Input: part model. Units: mm. Frame: model coordinates. A direction names the side the tool comes from. Give positions to 0.01 mm unless a question says otherwise; leave off trailing zeros. Order: outer loops, then holes, each group sorted by start corner. A loop starts at its lowest first (then second) coordinate and runs counter-clockwise, first axis right, second up. Notation, with made-up numbers: (11, 82) -> (68, 82) arc R20 ccw to (68, 106) -> close; hole circle Ø11 at (57.5, 73). An arc over 180 degrees is marked (long way). Use a Markdown table: item, result. Add a question column.
from build123d import *

# Parameters (mm, degrees)
SKETCH1_R           = 7.750000000000002
SKETCH1_R_2         = 2.7500000000000013
SKETCH1_R_3         = 7.749999999999997
SKETCH1_R_4         = 2.7499999999999973
BOSS_EXTRUDE1_DEPTH = 5
BOSS_EXTRUDE2_DEPTH = 5
BOSS_EXTRUDE3_DEPTH = 10
BOSS_EXTRUDE4_DEPTH = 5
FILLET1_R           = 5
SKETCH6_R           = 3.5
CUT_EXTRUDE1_DEPTH  = 5
CUT_EXTRUDE2_DEPTH  = 3
BOSS_EXTRUDE5_DEPTH = 3
FILLET2_R           = 10
BOSS_EXTRUDE6_DEPTH = 5
FILLET3_R           = 2


with BuildPart() as part:
    # Sketch1 → Boss-Extrude1 (new body)
    # profile 1 of 4: a face of its own
    with BuildSketch(Plane.XY):
        with BuildLine():
            ThreePointArc((-10.000000000000002, 33.49999999999998), (-17.75, 41.24999999999998), (-10, 48.99999999999998))
            Line((-10, 48.99999999999998), (-60.00000000000001, 48.99999999999998))
            Line((-60.00000000000001, 48.99999999999998), (-60, 33.49999999999997))
            Line((-60, 33.49999999999997), (-10, 33.49999999999998))
        make_face()
    # profile 2 of 4: a face of its own
    with BuildSketch(Plane.XY):
        with Locations((-10, 41.24999999999998)):
            Circle(SKETCH1_R)
        with Locations((-10, 41.24999999999998)):
            Circle(SKETCH1_R_2, mode=Mode.SUBTRACT)
    # profile 3 of 4: a face of its own
    with BuildSketch(Plane.XY):
        with Locations((-9.999999999999927, -41.24999999999999)):
            Circle(SKETCH1_R_3)
        with Locations((-9.999999999999927, -41.24999999999999)):
            Circle(SKETCH1_R_4, mode=Mode.SUBTRACT)
    # profile 4 of 4: a face of its own
    with BuildSketch(Plane.XY):
        with BuildLine():
            Line((-59.99999999999993, -48.999999999999986), (-9.999999999999927, -48.99999999999999))
            ThreePointArc((-9.999999999999929, -48.99999999999999), (-17.749999999999925, -41.24999999999999), (-9.999999999999927, -33.49999999999999))
            Line((-9.999999999999927, -33.49999999999999), (-59.99999999999993, -33.5))
            Line((-59.99999999999993, -33.5), (-59.99999999999993, -48.999999999999986))
        make_face()
    extrude(amount=BOSS_EXTRUDE1_DEPTH)

    # Sketch2 → Boss-Extrude2 (add)
    with BuildSketch(Plane.XY.offset(5)):
        Polygon((-53.500000000000014, -7.500000000000029), (-53.500000000000014, 7.499999999999971), (-53.500000000000014, 33.49999999999998), (-60, 33.49999999999997), (-59.99999999999993, -33.5), (-53.500000000000014, -33.49999999999999), align=None)
    extrude(amount=-BOSS_EXTRUDE2_DEPTH)

    # Sketch3 → Boss-Extrude3 (add)
    with BuildSketch(Plane.XY.offset(5)):
        Polygon((-59.99999999999997, -6.94e-15), (-53.500000000000014, 0), (-53.500000000000014, 10), (-59.99999999999997, 9.999999999999986), align=None)
        Polygon((-53.500000000000014, -10), (-53.500000000000014, 0), (-59.99999999999997, -6.94e-15), (-59.99999999999997, -10.000000000000014), align=None)
    extrude(amount=BOSS_EXTRUDE3_DEPTH)

    # Sketch4 → Boss-Extrude4 (add)
    with BuildSketch(Plane.XY.offset(15)):
        Polygon((-53.500000000000014, -10.000000000000007), (-53.500000000000014, 9.999999999999993), (-59.99999999999999, 9.999999999999986), (-59.99999999999998, -10.000000000000014), align=None)
    extrude(amount=BOSS_EXTRUDE4_DEPTH)

    # Fillet1
    fillet1_edges = [part.edges().sort_by_distance(p)[0] for p in [
        (-56.74999999999999, 9.999999999999993, 5),
        (-56.74999999999999, -10.000000000000007, 5),
        (-56.75, -10.00000000000001, 20),
        (-56.75, 9.99999999999999, 20),
    ]]
    fillet(fillet1_edges, radius=FILLET1_R)

    # Sketch6 → Cut-Extrude1 (cut)
    with BuildSketch(Plane(origin=(-53.500000000000014, 0, 0), x_dir=(0, 0, -1), z_dir=(1, -1e-16, 0))):
        with Locations(Location((-8.500000000000007, -3.49e-15, 0), (0, 0, 90))):
            Circle(SKETCH6_R)
    extrude(amount=-CUT_EXTRUDE1_DEPTH, mode=Mode.SUBTRACT)

    # Sketch7 → Cut-Extrude2 (cut)
    with BuildSketch(Plane.ZY.offset(59.999999999999986)):
        Polygon((8.500000000000009, -8.99999999999997), (8.500000000000007, 2.958e-14), (8.500000000000007, 9.000000000000028), (7.000000000000008, 9.000000000000028), (7.000000000000008, 2.958e-14), (7.000000000000008, -8.99999999999997), align=None)
        Polygon((8.500000000000007, 9.000000000000028), (8.500000000000007, 2.958e-14), (8.500000000000009, -8.99999999999997), (10.000000000000007, -8.99999999999997), (10.000000000000007, 2.958e-14), (10.000000000000007, 9.000000000000028), align=None)
        Polygon((8.500000000000007, 9.000000000000028), (8.500000000000007, 2.958e-14), (8.500000000000009, -8.99999999999997), (10.000000000000007, -8.99999999999997), (10.000000000000007, 2.958e-14), (10.000000000000007, 9.000000000000028), align=None)
        Polygon((8.500000000000009, -8.99999999999997), (8.500000000000007, 2.958e-14), (8.500000000000007, 9.000000000000028), (7.000000000000008, 9.000000000000028), (7.000000000000008, 2.958e-14), (7.000000000000008, -8.99999999999997), align=None)
    extrude(amount=-CUT_EXTRUDE2_DEPTH, mode=Mode.SUBTRACT)

    # Sketch9 → Boss-Extrude5 (add)
    with BuildSketch(Plane.ZY.offset(56.99999999999998)):
        with BuildLine():
            Line((7.000000000000008, -3.1622776601683573), (7.000000000000008, -8.999999999999968))
            Line((7.000000000000008, -8.999999999999968), (10.000000000000007, -8.999999999999968))
            Line((10.000000000000007, -8.999999999999968), (10.000000000000007, -3.1622776601683573))
            ThreePointArc((10.000000000000007, -3.1622776601683573), (8.500000000000007, -3.4999999999999774), (7.000000000000008, -3.1622776601683573))
        make_face()
    extrude(amount=BOSS_EXTRUDE5_DEPTH)

    # Fillet2
    fillet2_edges = [part.edges().sort_by_distance(p)[0] for p in [
        (-60.00000000000001, 48.99999999999998, 2.5),
        (-53.500000000000014, 33.49999999999998, 2.5),
        (-53.500000000000014, -33.49999999999999, 2.5),
        (-59.99999999999993, -48.999999999999986, 2.5),
    ]]
    fillet(fillet2_edges, radius=FILLET2_R)

    # Sketch10 → Boss-Extrude6 (add)
    with BuildSketch(Plane.ZY.offset(59.999999999999986)):
        Polygon((5, -14.999999999999988), (0, -14.999999999999986), (0, -38.99999999999997), (5, -38.999999999999964), align=None)
        Polygon((0, 15.000000000000014), (5.000000000000004, 15.000000000000012), (5, 39), (0, 39), align=None)
    extrude(amount=BOSS_EXTRUDE6_DEPTH)

    # Fillet3
    fillet3_edges = [part.edges().sort_by_distance(p)[0] for p in [
        (-59.99999999999993, 38.99999999999997, 2.5),
        (-59.99999999999993, -38.999999999999986, 2.5),
        (-59.99999999999998, -15.000000000000012, 2.5),
        (-64.99999999999999, -15.000000000000014, 2.5),
        (-64.99999999999997, -38.99999999999999, 2.5),
        (-64.99999999999999, 14.999999999999986, 2.500000000000002),
        (-65, 38.99999999999997, 2.5),
        (-59.99999999999999, 14.999999999999988, 2.500000000000002),
    ]]
    fillet(fillet3_edges, radius=FILLET3_R)


solid = part.part
Q1. First-contact query: pin 1 (6 mm diameter, centred on x = -56.5, y = -31.5, fed in from +Z); pin 2 (0.5 mm diameter, centred on x = -62.5, z = 3, fed in from -Y); pin 3 (6 mm diameter, centred on y = 3, z = 6.5, fed in from +X). Flat tips, straight axial feed; report the tip coordinate or a pass-through.
Q2. Access query for faces 5 (the cylindrical face through (-64.4, 15.57, 2.54)), 6 (the cylindrical face through (-55.982, -3.497, 8.654)), 7 (the flat face through (-59, 4, 10)), 8 (the flat face through (-27, 33.5, 2)). Directions: +Z, -Z, +X, -X, +Y, -Y. A direction counts if a zero-diameter tool reaches every point of the face in a straight line with its end or side. Return the directions, or none.
Q3. Section query C-C (y = 0). Return loops of the section in (x, z).
Q4. Draft query along Y for faces 1 (the flat face through (-40, -36, 5)), 2 (the flat face through (-60, 0, 12)), 3 (the flat face through (-58.5, 0, 11)), 4 (the cylindrical face through (-56.5, 46.6, 2.5)). Return one class per face: +Y half, -Y half, draft (parallel to the pull), parting line (faces both ways), or undercut.
Q5. Section query A-A (x = -23.5). Return loops of the section in (y, z), plus the area to 3 significant figures.
Q6. Ray query, line 1 (Z direction, x = -57.25, y = 0); line 2 (Z direction, x = -51, y = 40); line 3 (X direction, y = 3, z = 5.25). Return the intervals inside material, ascending.
Q7. Section query D-D (x = -48). Return loops of the section in (y, z).
Solution:
| question | item | result |
|---|---|---|
| 1 | pin 1 | stops at z = 5 |
| 1 | pin 2 | stops at y = -39 |
| 1 | pin 3 | stops at x = -53.5 |
| 2 | face 5 | +Z, -Z, -X |
| 2 | face 6 | +X |
| 2 | face 7 | -X |
| 2 | face 8 | +Z, -Z, +X |
| 3 | outline | (-60, 0) -> (-53.5, 0) -> (-53.5, 5) -> (-58.5, 5) -> (-58.5, 7) -> (-60, 7) -> close; (-60, 10) -> (-58.5, 10) -> (-58.5, 12) -> (-53.5, 12) -> (-53.5, 20) -> (-60, 20) -> close |
| 4 | face 1 | draft |
| 4 | face 2 | undercut |
| 4 | face 3 | undercut |
| 4 | face 4 | +Y half |
| 5 | outline | (-49, 0) -> (-33.5, 0) -> (-33.5, 5) -> (-49, 5) -> close; (33.5, 0) -> (49, 0) -> (49, 5) -> (33.5, 5) -> close |
| 5 | area | 155 mm² |
| 6 | line 1 | z = 0 to 5, 12 to 20 |
| 6 | line 2 | z = 0 to 5 |
| 6 | line 3 | x = -60 to -53.5 |
| 7 | outline | (-49, 0) -> (-32.43, 0) -> (-32.43, 5) -> (-49, 5) -> close; (32.43, 0) -> (49, 0) -> (49, 5) -> (32.43, 5) -> close |
